```python
from build123d import *

# Parameters (mm, degrees)
F0_W     = 101.6
F0_H     = 101.6
F1_DEPTH = 101.6
F2_R     = 20.257871
F3_DEPTH = 101.601
F4_R     = 15.235022
F5_DEPTH = 101.601


with BuildPart() as f1:
    # F0 (on Front) → F1 (new body)
    with BuildSketch(Plane.XZ):
        with Locations((-4.734128, 2.650937)):
            Rectangle(F0_W, F0_H)
    extrude(amount=F1_DEPTH)

    # F2 (on face) → F3 (cut, through all)
    with BuildSketch(Plane.XZ.offset(101.6)):
        with Locations((-23.539765, 27.651252)):
            Circle(F2_R)
    extrude(amount=-F3_DEPTH, mode=Mode.SUBTRACT)

    # F4 (on face) → F5 (intersect, through all)
    with BuildSketch(Plane(origin=(-55.534128, 0, 0), x_dir=(0, -1, 0), z_dir=(-1, 0, 0))):
        with Locations((48.238128, 36.392964)):
            Circle(F4_R)
    extrude(amount=-F5_DEPTH, mode=Mode.INTERSECT)


solid = f1.part
```
Source: CAD feature listing. Evaluate the final solid. Frame: model axes, mm. Round coordinates to 2 decimals unless told otherwise and drop trailing zeros. Loops run counter-clockwise (first coordinate to the right, second up) from the corner with the lowest first, then second, coordinate; pieces in that order, holes last. Notation, with made-up numbers: M 18,5.5 L 23,5.5 A20 cw 23,42.5 Z; hole C 45,32.25 d10. An arc over 180 degrees is marked long. Use a Markdown table: item, result. Add a question column.
1. Line query: line 1 (X direction, y = -59.5, z = 27.5); line 2 (X direction, y = -56.5, z = 25); line 3 (Y direction, x = 30.5, z = 37). Output: solid intervals per line, ascending.
2. Section query C-C on y = -55. Return the cut outline in (x, z).
3. Section query B-B on y = -60. Return the cut outline in (x, z).
4. Contact query for flat-ended pins moving along their axis: P1, Ø6, axis at x = -33.5, y = -60, coming from the +Z side; P2, Ø1.5, axis at x = -5.5, z = 41.5, coming from the -Y side; P3, Ø12, axis at x = 16.5, z = 25.5, coming from the -Y side. Output: stop coordinate, or through.
5. Mould query, pull axis Z, two halves, no side actions, for faces 1 (the cylindrical face through (5.844, -46.255, 51.498)), 2 (the flat face through (-55.534, -48, 37)), 3 (the cylindrical face through (-23, -48.5, 47.9)). Classes: pulls with the +Z half, pulls with the -Z half, needs draft (parallel to the pull), parting line crosses it, or undercut.
6. Section query A-A on z = 45.5. Return the cut outline in (x, y).
7. Section query D-D on x = 36. Return the cut outline in (y, z), then the cut area to 3 significant figures.
Reported:
| question | item | result |
|---|---|---|
| 1 | line 1 | x = -55.53 to -43.8, -3.28 to 46.07 |
| 1 | line 2 | x = -55.53 to -43.62, -3.46 to 46.07 |
| 1 | line 3 | y = -63.46 to -33.02 |
| 2 | outline | M -55.53,22.74 L -43.19,22.74 A20.26 cw long -3.89,22.74 L 46.07,22.74 L 46.07,50.05 L -55.53,50.05 Z |
| 3 | outline | M -55.53,26.71 L -43.78,26.71 A20.26 cw -31.96,46.08 L -55.53,46.08 Z; M -15.12,46.08 A20.26 cw -3.3,26.71 L 46.07,26.71 L 46.07,46.08 Z |
| 4 | P1 | stops at z = 48.86 |
| 4 | P2 | stops at y = -62.84 |
| 4 | P3 | stops at y = -62.67 |
| 5 | face 1 | parting line crosses it |
| 5 | face 2 | needs draft |
| 5 | face 3 | undercut |
| 6 | outline | M -55.53,-60.45 L -33.12,-60.45 L -33.12,-36.02 L -55.53,-36.02 Z; M -13.96,-60.45 L 46.07,-60.45 L 46.07,-36.02 L -13.96,-36.02 Z |
| 7 | outline | C -48.24,36.39 d30.47 |
| 7 | area | 729 mm² |
